from build123d import *

# Parameters (mm, degrees)
F0_W     = 101.6
F0_H     = 146.05
F1_DEPTH = 3.175
F2_W     = 3.175
F2_H     = 25.4
F3_DEPTH = 3.175
F4_W     = 25.4
F4_H     = 3.175
F5_DEPTH = 3.175


with BuildPart() as f1:
    # F0 (on Top) → F1 (new body)
    with BuildSketch(Plane.XY):
        Rectangle(F0_W, F0_H)
    extrude(amount=F1_DEPTH)

    # F2 (on Top) → F3 (cut)
    with BuildSketch(Plane.XY):
        with Locations((-49.2125, 0)):
            Rectangle(F2_W, F2_H)
        with Locations((49.2125, 0)):
            Rectangle(F2_W, F2_H)
    extrude(amount=F3_DEPTH, mode=Mode.SUBTRACT)

    # F4 (on Top) → F5 (join)
    with BuildSketch(Plane.XY):
        with Locations((0, 74.6125)):
            Rectangle(F4_W, F4_H)
        with Locations((0, -74.6125)):
            Rectangle(F4_W, F4_H)
    extrude(amount=F5_DEPTH)


solid = f1.part
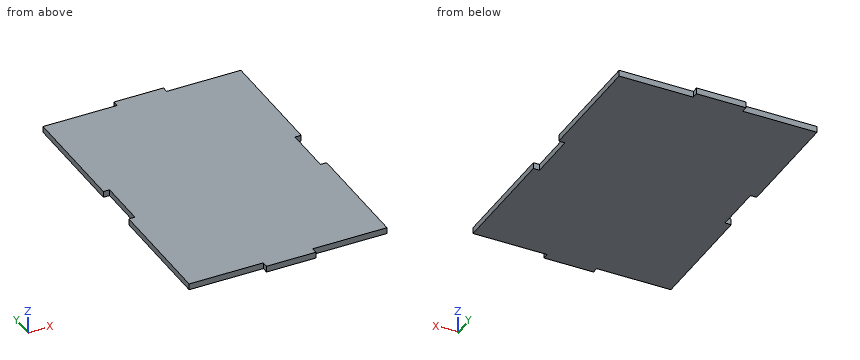
Part model, mm, in its own coordinate system. Round coordinates to 2 decimals unless told otherwise and drop trailing zeros. Write each loop counter-clockwise with the first axis right and the second up, starting at its lowest first coordinate (ties: lowest second). Pieces come first, ordered by that corner, then holes. Notation, with made-up numbers: M 86,27 L 117,27 A30 cw 117,59 Z; hole C 6.25,0.5 d6. An arc over 180 degrees is marked long. Return JSON: item names as keys, results as strings. Group by question number.
(1) Drill centre lines: probe 1 along X at (y, z) = (8, 2.85) (3 decimals); probe 2 along Y at (x, z) = (39.5, 2.8) (3 decimals). Where is each one in solid material? Low to high.
(2) Pin check, flat tips, straight feed: pin 1 Ø1 at (x, z) = (48.5, 2) entering from -Y (3 decimals); pin 2 Ø1 at (y, z) = (-75, 1.5) entering from -X; pin 3 Ø1.6 at (x, z) = (-50, 1.5) entering from +Y (3 decimals). Stop position of each tip, or through.
(3) Saw through at A-A on z = 1.3. Write the cut outline in (x, y) (3 decimals).
(4) Saw through at B-B on x = 15. Write the cut outline in (y, z) (3 decimals), then the cut area to 3 significant figures.
(5) Saw through at C-C on y = -10.5. Write the cut outline in (x, z) (3 decimals).
Returned:
{
 "1": {"probe 1": "-47.625 to 47.625", "probe 2": "-73.025 to 73.025"},
 "2": {"pin 1": "y = -73.025", "pin 2": "x = -12.7", "pin 3": "y = 73.025"},
 "3": {"outline": "M -50.8,-73.025 L -12.7,-73.025 L -12.7,-76.2 L 12.7,-76.2 L 12.7,-73.025 L 50.8,-73.025 L 50.8,-12.7 L 47.625,-12.7 L 47.625,12.7 L 50.8,12.7 L 50.8,73.025 L 12.7,73.025 L 12.7,76.2 L -12.7,76.2 L -12.7,73.025 L -50.8,73.025 L -50.8,12.7 L -47.625,12.7 L -47.625,-12.7 L -50.8,-12.7 Z"},
 "4": {"outline": "M -73.025,0 L 73.025,0 L 73.025,3.175 L -73.025,3.175 Z", "area": "464 mm²"},
 "5": {"outline": "M -47.625,0 L 47.625,0 L 47.625,3.175 L -47.625,3.175 Z"}
}
